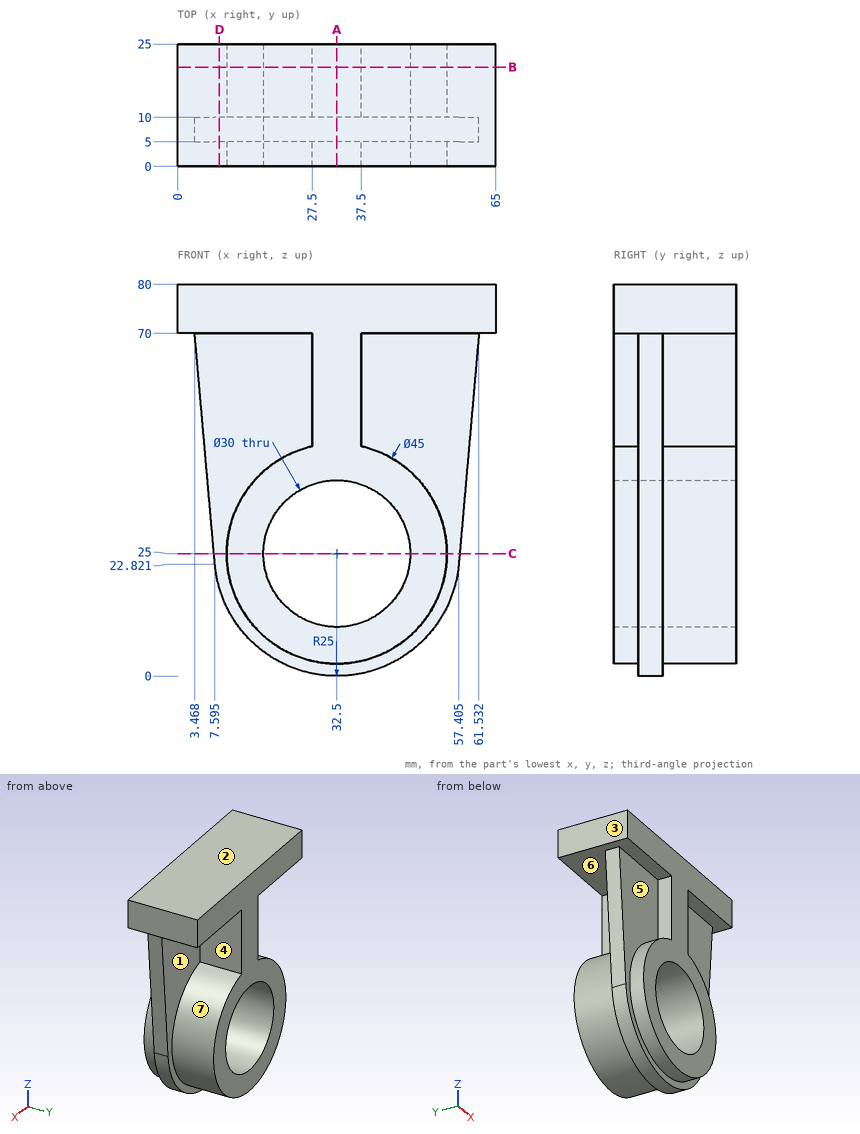
The drawing under review shows one solid part. Ordinate dimensions are in mm from its lowest x, y, z. A direction names the side the tool comes from. Round coordinates to 2 decimals unless told otherwise and drop trailing zeros. Write each loop counter-clockwise with the first axis right and the second up, starting at its lowest first coordinate (ties: lowest second). Pieces come first, ordered by that corner, then holes. Notation, with made-up numbers: (85.5, 34.5) -> (122.5, 34.5) arc R11 ccw to (122.5, 44.5) -> close; hole circle Ø10 at (28, 11.5). An arc over 180 degrees is marked (long way). One line per question, with ' | ' between items. Start each with the question number.
(1) Add section D-D, the plane x = 8.5. Write out the cut boundary in (y, z), plus the area to 3 significant figures.
(2) Tool access review of the marked faces 4, 5, 6 and 7: name each direction out of +Z, -Z, +X, -X, +Y, -Y from which nothing blocks a thin tool from reaching the whole face with its end or side.
(3) For line 1 along X through (y, z) = (19.5, 25); line 2 along Z through (x, y) = (23.5, 4.25); line 3 along X through (y, z) = (16.5, 52.5), list the stretches that pass through material, from the lowest coordinate up. Write a range as from..to.
(4) Insertion check: P1, Ø5.5, axis at y = 2, z = 55, coming from the +X side; P2, Ø1, axis at x = 7, z = 35.5, coming from the -Y side; P3, Ø7.5, axis at x = 9, y = 8.5, coming from the -Z side. Each pin has a flat end and moves straight along its axis. Give the tip position at first contact, or say it passes through.
(5) Add section B-B, the plane y = 20.25. Write out the cut boundary in (x, z), plus the area to 3 significant figures.
(6) Mouldability with a two-part tool opening along Z and no side actions: class the marked faces 1, 2 and 3 as released by +Z, released by -Z, zero draft, split by the parting line, or undercut.
(7) Add section A-A, the plane x = 32.5. Write out the cut boundary in (y, z), plus the area to 3 significant figures.
(8) Add section C-C, the plane z = 25. Write out the cut boundary in (x, y) (1 decimal).
Answer list:
1) outline: (0, 70) -> (5, 70) -> (5, 18) -> (10, 18) -> (10, 70) -> (25, 70) -> (25, 80) -> (0, 80) -> close | area: 510 mm²
2) face 4: +X, +Y | face 5: -Y | face 6: -X | face 7: +Y
3) line 1: 10..17.5, 47.5..55 | line 2: 4.38..13, 37..45.62, 70..80 | line 3: 27.5..37.5
4) P1: x = 37.5 | P2: y = 5 | P3: z = 9.67
5) outline: (0, 70) -> (27.5, 70) -> (27.5, 46.94) arc R22.5 ccw (long way) to (37.5, 46.94) -> (37.5, 70) -> (65, 70) -> (65, 80) -> (0, 80) -> close; hole circle Ø30 at (32.5, 25) | area: 1,760 mm²
6) face 1: undercut | face 2: released by +Z | face 3: zero draft
7) outline: (0, 2.5) -> (5, 2.5) -> (5, 0) -> (10, 0) -> (10, 2.5) -> (25, 2.5) -> (25, 10) -> (0, 10) -> close; (0, 40) -> (25, 40) -> (25, 80) -> (0, 80) -> close | area: 1,200 mm²
8) outline: (7.4, 5) -> (10, 5) -> (10, 0) -> (17.5, 0) -> (17.5, 25) -> (10, 25) -> (10, 10) -> (7.4, 10) -> close; (47.5, 0) -> (55, 0) -> (55, 5) -> (57.6, 5) -> (57.6, 10) -> (55, 10) -> (55, 25) -> (47.5, 25) -> close
